from build123d import *

# Parameters (mm, degrees)
SKETCH_1_W          = 12
SKETCH_1_H          = 12
EXTRUDE_1_DEPTH     = 9.64
SKETCH_2_R          = 5.5
EXTRUDE_2_DEPTH     = 74.3
SKETCH_3_W          = 12
SKETCH_3_H          = 12
EXTRUDE_3_DEPTH     = 12.55
SKETCH_4_R          = 4
EXTRUDE_4_DEPTH     = 8
SKETCH_5_R          = 2.1
CUT_EXTRUDE_1_DEPTH = 94
SKETCH_6_R          = 10.507277245
SKETCH_6_R_2        = 7
CUT_EXTRUDE_2_DEPTH = 102
SKETCH_7_R          = 2
CUT_EXTRUDE_3_DEPTH = 6


with BuildPart() as part:
    # Sketch 1 → Extrude 1 (new body)
    with BuildSketch(Plane(origin=(0, 0, 0), x_dir=(1, 0, 0), z_dir=(0, 1, 0))):
        Rectangle(SKETCH_1_W, SKETCH_1_H)
    extrude(amount=EXTRUDE_1_DEPTH)

    # Sketch 2 → Extrude 2 (add)
    with BuildSketch(Plane(origin=(0, 9.64, 0), x_dir=(1, 0, 0), z_dir=(0, 1, 0))):
        with Locations(Location((0, 0, 0), (0, 0, 270))):
            Circle(SKETCH_2_R)
    extrude(amount=EXTRUDE_2_DEPTH)

    # Sketch 3 → Extrude 3 (add)
    with BuildSketch(Plane(origin=(0, 83.94, 0), x_dir=(1, 0, 0), z_dir=(0, 1, 0))):
        Rectangle(SKETCH_3_W, SKETCH_3_H)
    extrude(amount=EXTRUDE_3_DEPTH)

    # Sketch 4 → Extrude 4 (add)
    with BuildSketch(Plane(origin=(0, 96.49, 0), x_dir=(1, 0, 0), z_dir=(0, 1, 0))):
        with Locations(Location((0, 0, 0), (0, 0, 270))):
            Circle(SKETCH_4_R)
    extrude(amount=EXTRUDE_4_DEPTH)

    # Sketch 5 → Cut-Extrude 1 (cut)
    with BuildSketch(Plane(origin=(0, 104.49, 0), x_dir=(1, 0, 0), z_dir=(0, 1, 0))):
        with Locations(Location((0, 0, 0), (0, 0, 270))):
            Circle(SKETCH_5_R)
    extrude(amount=-CUT_EXTRUDE_1_DEPTH, mode=Mode.SUBTRACT)

    # Sketch 6 → Cut-Extrude 2 (cut)
    with BuildSketch(Plane(origin=(0, 96.49, 0), x_dir=(1, 0, 0), z_dir=(0, 1, 0))):
        Circle(SKETCH_6_R)
        Circle(SKETCH_6_R_2, mode=Mode.SUBTRACT)
    extrude(amount=-CUT_EXTRUDE_2_DEPTH, mode=Mode.SUBTRACT)

    # Sketch 7 → Cut-Extrude 3 (cut)
    with BuildSketch(Plane(origin=(6, 0, 0), x_dir=(0, 0, -1), z_dir=(1, 0, 0))):
        with Locations((0, 4)):
            Circle(SKETCH_7_R)
        with Locations((0, 89.44)):
            Circle(SKETCH_7_R)
    extrude(amount=-CUT_EXTRUDE_3_DEPTH, mode=Mode.SUBTRACT)


solid = part.part
The model under review builds one solid part; all positions refer to its coordinate system, in mm. A direction names the side the tool comes from. Round coordinates to 2 decimals unless told otherwise and drop trailing zeros. Loops run counter-clockwise (first coordinate to the right, second up) from the corner with the lowest first, then second, coordinate; pieces in that order, holes last. Notation, with made-up numbers: (-18.5, -0.75) -> (24.5, -0.75) arc R7 ccw to (24.5, 9.25) -> close; hole circle Ø1 at (12, -36). An arc over 180 degrees is marked (long way). Return JSON: item names as keys, results as strings.
(1) Add section C-C on y = 21. Write out the cut boundary in (x, z).
Solved:
{"outline": "circle Ø11 at (0, 0); hole circle Ø4.2 at (0, 0)"}
(2) For line 1 (Y direction, x = 3.35, z = 0); line 2 (X direction, y = 34, z = 0); line 3 (Z direction, x = 2.55, y = 89.44), list the stretches that pass through material, from the lowest coordinate up.
Solved:
{"line 1": "0 to 2, 6 to 87.44, 91.44 to 104.49", "line 2": "-5.5 to -2.1, 2.1 to 5.5", "line 3": "-6 to -2, 2 to 6"}
(3) For faces 4 (the flat face through (-4.1, 96.49, -1.4)), 5 (the flat face through (0, 90, -6)), 6 (the cylindrical face through (3, 2, 0)), list the 3-axis set-ups (+Z, -Z, +X, -X, +Y, -Y) from which the entire face can be reached by the end or side of a thin tool; tool diameter is ignored.
Solved:
{"face 4": "+Y", "face 5": "-Z, +X, -X, +Y, -Y", "face 6": "+X"}
(4) For pin 1 (3 mm diameter, centred on y = 66.5, z = -4.5, fed in from -X); pin 2 (1.2 mm diameter, centred on y = 3.5, z = -1, fed in from +X); pin 3 (5 mm diameter, centred on y = 25.5, z = -1.5, fed in from -X), all flat-tipped, find the tip position at first contact; note any pin that passes through.
Solved:
{"pin 1": "x = -4.61", "pin 2": "x = 0", "pin 3": "x = -5.5"}
(5) Add section B-B on y = 92.5. Write out the cut boundary in (x, z), plus the area to 3 significant figures.
Solved:
{"outline": "(-6, -3.61) arc R7 ccw to (-3.61, -6) -> (3.61, -6) arc R7 ccw to (6, -3.61) -> (6, 3.61) arc R7 ccw to (3.61, 6) -> (-3.61, 6) arc R7 ccw to (-6, 3.61) -> close; hole circle Ø4.2 at (0, 0)", "area": "121 mm2"}
(6) The part is to be moulded in two halves that separate along X. For faces 1 (the flat face through (0, 10.49, 0)), 2 (the flat face through (-6, 90, 0)), 3 (the flat face through (-2, 104.49, 2)), say which applies: released by +X, released by -X, zero draft, split by the parting line, or undercut.
Solved:
{"face 1": "undercut", "face 2": "released by -X", "face 3": "zero draft"}
(7) Add section A-A on z = 0. Write out the cut boundary in (x, y), plus the area to 3 significant figures.
Solved:
{"outline": "(-6, 0) -> (6, 0) -> (6, 2) -> (0, 2) -> (0, 6) -> (6, 6) -> (6, 9.64) -> (5.5, 9.64) -> (5.5, 83.94) -> (6, 83.94) -> (6, 87.44) -> (2.1, 87.44) -> (2.1, 10.49) -> (-2.1, 10.49) -> (-2.1, 104.49) -> (-4, 104.49) -> (-4, 96.49) -> (-6, 96.49) -> (-6, 83.94) -> (-5.5, 83.94) -> (-5.5, 9.64) -> (-6, 9.64) -> close; (2.1, 91.44) -> (6, 91.44) -> (6, 96.49) -> (4, 96.49) -> (4, 104.49) -> (2.1, 104.49) -> close", "area": "713 mm2"}
